CAD build for the part. Positions are in the model's coordinates, mm. A direction names the side the tool comes from. Give positions to 0.01 mm unless a question says otherwise; leave off trailing zeros. Loops run counter-clockwise (first coordinate to the right, second up) from the corner with the lowest first, then second, coordinate; pieces in that order, holes last.
```python
from build123d import *

# Parameters (mm, degrees)
SKETCH_1_R      = 1.5
SKETCH_1_R_2    = 9.5
SKETCH_1_W      = 10
SKETCH_1_H      = 15
SKETCH_1_R_3    = 1.3
SKETCH_1_W_2    = 20
SKETCH_1_H_2    = 20
EXTRUDE_1_DEPTH = 5
FILLET_1_R      = 7
FILLET_2_R      = 10


with BuildPart() as part:
    # 草图1 → 凸台-拉伸1 (new body)
    with BuildSketch(Plane(origin=(0, 0, 0), x_dir=(1, 0, 0), z_dir=(0, 1, 0))):
        with BuildLine():
            Line((160, 0), (0, 0))
            Line((0, 0), (0, -91))
            Line((0, -91), (-15.211013308, -91))
            ThreePointArc((-15.211013308, -91), (-14.22252688, -91.790417714), (-13.85, -93))
            ThreePointArc((-13.85, -93), (-17.209582286, -94.77747312), (-16.788986692, -91))
            Line((-16.788986692, -91), (-25.211013308, -91))
            ThreePointArc((-25.211013308, -91), (-24.22252688, -91.790417714), (-23.85, -93))
            ThreePointArc((-23.85, -93), (-27.209582286, -94.77747312), (-26.788986692, -91))
            Line((-26.788986692, -91), (-50, -91))
            Line((-50, -91), (-50, -159))
            Line((-50, -159), (0, -159))
            Line((0, -159), (0, -250))
            Line((0, -250), (160, -250))
            Line((160, -250), (160, -167.5))
            ThreePointArc((160, -167.5), (149.692235936, -166.231056256), (140, -162.5))
            Line((140, -162.5), (100, -162.5))
            Line((100, -162.5), (100, -87.5))
            Line((100, -87.5), (140, -87.5))
            ThreePointArc((140, -87.5), (149.692235936, -83.768943744), (160, -82.5))
            Line((160, -82.5), (160, 0))
        make_face()
        with Locations(Location((6, -244, 0), (0, 0, 270))):
            Circle(SKETCH_1_R, mode=Mode.SUBTRACT)
        with Locations(Location((20, -165, 0), (0, 0, 270))):
            Circle(SKETCH_1_R, mode=Mode.SUBTRACT)
        with Locations(Location((50, -165, 0), (0, 0, 270))):
            Circle(SKETCH_1_R, mode=Mode.SUBTRACT)
        with Locations(Location((70.5, -220, 0), (0, 0, 270))):
            Circle(SKETCH_1_R_2, mode=Mode.SUBTRACT)
        with Locations(Location((105, -230, 0), (0, 0, 270))):
            Circle(SKETCH_1_R, mode=Mode.SUBTRACT)
        with Locations((80, -192.5)):
            Rectangle(SKETCH_1_W, SKETCH_1_H, mode=Mode.SUBTRACT)
        with Locations(Location((105, -192.5, 0), (0, 0, 270))):
            Circle(SKETCH_1_R, mode=Mode.SUBTRACT)
        with Locations(Location((116.5, -223.25, 0), (0, 0, 270))):
            Circle(SKETCH_1_R_3, mode=Mode.SUBTRACT)
        with Locations(Location((125, -230, 0), (0, 0, 270))):
            Circle(SKETCH_1_R, mode=Mode.SUBTRACT)
        with Locations(Location((154, -244, 0), (0, 0, 270))):
            Circle(SKETCH_1_R, mode=Mode.SUBTRACT)
        with Locations(Location((143, -223.25, 0), (0, 0, 270))):
            Circle(SKETCH_1_R_3, mode=Mode.SUBTRACT)
        with Locations(Location((116.5, -199.25, 0), (0, 0, 270))):
            Circle(SKETCH_1_R_3, mode=Mode.SUBTRACT)
        with Locations(Location((125, -192.5, 0), (0, 0, 270))):
            Circle(SKETCH_1_R, mode=Mode.SUBTRACT)
        with Locations(Location((143, -199.25, 0), (0, 0, 270))):
            Circle(SKETCH_1_R_3, mode=Mode.SUBTRACT)
        with Locations(Location((152, -177, 0), (0, 0, 270))):
            Circle(SKETCH_1_R, mode=Mode.SUBTRACT)
        with BuildLine():
            Line((-31, -137), (-31, -97))
            Line((-31, -97), (-11, -97))
            Line((-11, -97), (-11, -137))
            Line((-11, -137), (-16, -137))
            Line((-16, -137), (-16, -138.85))
            ThreePointArc((-16, -138.85), (-13.85, -141), (-16, -143.15))
            Line((-16, -143.15), (-26, -143.15))
            ThreePointArc((-26, -143.15), (-28.15, -141), (-26, -138.85))
            Line((-26, -138.85), (-26, -137))
            Line((-26, -137), (-31, -137))
        make_face(mode=Mode.SUBTRACT)
        with Locations(Location((20, -85, 0), (0, 0, 270))):
            Circle(SKETCH_1_R, mode=Mode.SUBTRACT)
        with Locations(Location((50, -85, 0), (0, 0, 270))):
            Circle(SKETCH_1_R, mode=Mode.SUBTRACT)
        with Locations((47, -43)):
            Rectangle(SKETCH_1_W_2, SKETCH_1_H_2, mode=Mode.SUBTRACT)
        with Locations(Location((6, -6, 0), (0, 0, 270))):
            Circle(SKETCH_1_R, mode=Mode.SUBTRACT)
        with Locations(Location((152, -73, 0), (0, 0, 270))):
            Circle(SKETCH_1_R, mode=Mode.SUBTRACT)
        with Locations(Location((77, -61, 0), (0, 0, 270))):
            Circle(SKETCH_1_R, mode=Mode.SUBTRACT)
        with Locations(Location((77, -25, 0), (0, 0, 270))):
            Circle(SKETCH_1_R, mode=Mode.SUBTRACT)
        with Locations(Location((145, -61, 0), (0, 0, 270))):
            Circle(SKETCH_1_R, mode=Mode.SUBTRACT)
        with Locations(Location((145, -25, 0), (0, 0, 270))):
            Circle(SKETCH_1_R, mode=Mode.SUBTRACT)
        with Locations(Location((154, -6, 0), (0, 0, 270))):
            Circle(SKETCH_1_R, mode=Mode.SUBTRACT)
    extrude(amount=EXTRUDE_1_DEPTH)

    # 圆角1
    fillet_1_edges = [part.edges().sort_by_distance(p)[0] for p in [
        (0, 2.5, 91),
        (0, 2.5, 0),
        (160, 2.5, 0),
        (160, 2.5, 250),
        (0, 2.5, 250),
        (0, 2.5, 159),
        (-50, 2.5, 159),
        (-50, 2.5, 91),
    ]]
    fillet(fillet_1_edges, radius=FILLET_1_R)

    # 圆角2
    fillet_2_edges = [part.edges().sort_by_distance(p)[0] for p in [
        (160, 2.5, 82.5),
        (140, 2.5, 87.5),
        (100, 2.5, 87.5),
        (100, 2.5, 162.5),
        (140, 2.5, 162.5),
        (160, 2.5, 167.5),
    ]]
    fillet(fillet_2_edges, radius=FILLET_2_R)


solid = part.part
```
1. Probe line 1 along Z through (x, y) = (116.5, 2.45); line 2 along X through (y, z) = (1.75, 61); line 3 along Z through (x, y) = (132.5, 1.3). List the from-to ranges inside material, lowest first.
Responses:
line 1: z = 0 to 87.5, 162.5 to 197.95, 200.55 to 221.95, 224.55 to 250
line 2: x = 0 to 75.5, 78.5 to 143.5, 146.5 to 160
line 3: z = 0 to 87.5, 162.5 to 250
2. Saw through at C-C, the plane z = 203.5. List the corners of the cut face in (x, y), and give its area (3 significant figures).
Responses:
outline: (0, 0) - (160, 0) - (160, 5) - (0, 5) - close
area: 800 mm2
3. Tool access for faces 5 (the face through (0, 2, 204)), 6 (the face through (0, 2, 45)), 7 (the face through (146.87, 2.46, 165.42)), 8 (the face through (80, 2, 185)): list every direction of +Z, -Z, +X, -X, +Y, -Y with a clear straight run to the whole face (end or side of a thin tool).
Responses:
face 5: +Z, -X, +Y, -Y
face 6: -Z, -X, +Y, -Y
face 7: +X, +Y, -Y
face 8: +Y, -Y
4. Drop flat-ended pins along their axis: pin 1 (3 mm diameter, centred on y = 1, z = 191, fed in from -X); pin 2 (1.5 mm diameter, centred on x = -21, y = 3, fed in from -Z). Give the stop position or say it passes through.
Responses:
pin 1: stops at x = 0
pin 2: stops at z = 91
5. Pull direction Z, two halves, no side cores. Call faces 1 (the face through (-21, 2, 91)), 2 (the face through (102.85, 2.54, 159.49)), 3 (the face through (37, 2, 43)), 4 (the face through (-2, 2.5, 161.1)): released by +Z, released by -Z, zero draft, split by the parting line, or undercut.
Responses:
face 1: released by -Z
face 2: undercut
face 3: undercut
face 4: released by +Z
6. Saw through at A-A, the plane x = 70.5. List the corners of the cut face in (y, z), and give its area (4 significant figures).
Responses:
outline: (0, 0) - (5, 0) - (5, 210.5) - (0, 210.5) - close; (0, 229.5) - (5, 229.5) - (5, 250) - (0, 250) - close
area: 1,155 mm2
7. Saw through at B-B, the plane y = 3.75. Count the separate pieces of the cut face and the enclosed holes in it, and give its area (3 significant figures).
Responses:
separate pieces: 1
enclosed holes: 26
area: 36,800 mm2
